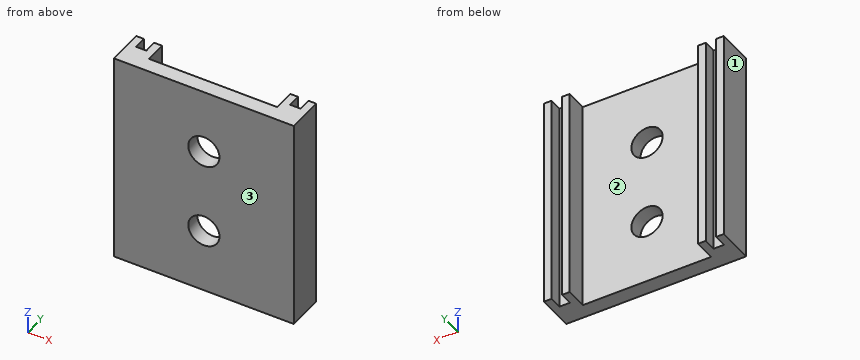
```python
from build123d import *

# Parameters (mm, degrees)
SKETCH1_W               = 40
SKETCH1_H               = 50
BOSS_EXTRUDE1_DEPTH     = 3.5
SKETCH2_W               = 40
SKETCH2_H               = 4
BOSS_EXTRUDE2_DEPTH     = 5
SKETCH3_W               = 4
SKETCH3_H               = 46
BOSS_EXTRUDE3_DEPTH     = 5
SKETCH4_W               = 2.4
SKETCH4_H               = 50
CUT_EXTRUDE1_DEPTH      = 3
SKETCH18_W              = 50
SKETCH18_H              = 8.5
BOSS_EXTRUDE8_DEPTH     = 1
SKETCH19_R              = 3.65
CUT_EXTRUDE2_DEPTH      = 6
CUT_EXTRUDE2_DEPTH_BACK = 4.5
SKETCH20_W              = 32
SKETCH20_H              = 4
CUT_EXTRUDE3_DEPTH      = 5
SKETCH21_W              = 50
SKETCH21_H              = 5
BOSS_EXTRUDE9_DEPTH     = 1


with BuildPart() as part:
    # Sketch1 → Boss-Extrude1 (new body)
    with BuildSketch(Plane(origin=(0, 0, 0), x_dir=(1, 0, 0), z_dir=(0, 1, 0))):
        Rectangle(SKETCH1_W, SKETCH1_H)
    extrude(amount=BOSS_EXTRUDE1_DEPTH)

    # Sketch2 → Boss-Extrude2 (add)
    with BuildSketch(Plane(origin=(0, 3.5, 0), x_dir=(1, 0, 0), z_dir=(0, 1, 0))):
        with Locations((0, 23)):
            Rectangle(SKETCH2_W, SKETCH2_H)
    extrude(amount=BOSS_EXTRUDE2_DEPTH)

    # Sketch3 → Boss-Extrude3 (add)
    with BuildSketch(Plane(origin=(0, 3.5, 0), x_dir=(1, 0, 0), z_dir=(0, 1, 0))):
        with Locations((-18, -2)):
            Rectangle(SKETCH3_W, SKETCH3_H)
    boss_extrude3 = extrude(amount=BOSS_EXTRUDE3_DEPTH)

    # Sketch4 → Cut-Extrude1 (cut)
    with BuildSketch(Plane(origin=(0, 8.5, 0), x_dir=(1, 0, 0), z_dir=(0, 1, 0))):
        with Locations((-18, 0)):
            Rectangle(SKETCH4_W, SKETCH4_H)
    cut_extrude1 = extrude(amount=-CUT_EXTRUDE1_DEPTH, mode=Mode.SUBTRACT)

    # Mirror1: Boss-Extrude3, Cut-Extrude1 across plane
    add(boss_extrude3.mirror(Plane(origin=(0, 0, 0), x_dir=(0, 0, 1), z_dir=(1, 0, 0))))
    add(cut_extrude1.mirror(Plane(origin=(0, 0, 0), x_dir=(0, 0, 1), z_dir=(1, 0, 0))), mode=Mode.SUBTRACT)

    # Sketch18 → Boss-Extrude8 (add)
    with BuildSketch(Plane.ZY.offset(20)):
        with Locations((0, 4.25)):
            Rectangle(SKETCH18_W, SKETCH18_H)
    boss_extrude8 = extrude(amount=BOSS_EXTRUDE8_DEPTH)

    # Mirror5: Boss-Extrude8 across plane
    add(boss_extrude8.mirror(Plane(origin=(0, 0, 0), x_dir=(0, 0, 1), z_dir=(1, 0, 0))))

    # Sketch19 → Cut-Extrude2 (cut, two sides)
    with BuildSketch(Plane(origin=(0, 3.5, 0), x_dir=(1, 0, 0), z_dir=(0, 1, 0))) as cut_extrude2_sk:
        with Locations((0, -10)):
            Circle(SKETCH19_R)
        with Locations((0, 10)):
            Circle(SKETCH19_R)
    extrude(amount=CUT_EXTRUDE2_DEPTH, mode=Mode.SUBTRACT)
    extrude(cut_extrude2_sk.sketch, amount=-CUT_EXTRUDE2_DEPTH_BACK, mode=Mode.SUBTRACT)

    # Sketch20 → Cut-Extrude3 (cut)
    with BuildSketch(Plane(origin=(0, 8.5, 0), x_dir=(1, 0, 0), z_dir=(0, 1, 0))):
        with Locations((0, 23)):
            Rectangle(SKETCH20_W, SKETCH20_H)
    extrude(amount=-CUT_EXTRUDE3_DEPTH, mode=Mode.SUBTRACT)

    # Sketch21 → Boss-Extrude9 (add)
    with BuildSketch(Plane(origin=(-16, 0, 0), x_dir=(0, 0, -1), z_dir=(1, 0, 0))):
        with Locations((0, 6)):
            Rectangle(SKETCH21_W, SKETCH21_H)
    boss_extrude9 = extrude(amount=BOSS_EXTRUDE9_DEPTH)

    # Mirror6: Boss-Extrude9 across plane
    add(boss_extrude9.mirror(Plane(origin=(0, 0, 0), x_dir=(0, 0, 1), z_dir=(1, 0, 0))))


solid = part.part
```
Check sheet for the modelled part. Datum: model origin and axes. Units: mm. Face numbers are marked on the shaded views. Coordinates: 2 decimals unless noted, no trailing zeros. Write each loop counter-clockwise with the first axis right and the second up, starting at its lowest first coordinate (ties: lowest second). Pieces come first, ordered by that corner, then holes. Notation, with made-up numbers: M 21.5,-7.75 L 43.5,-7.75 A31 ccw 43.5,25.25 Z; hole C 5.5,21.5 d11. An arc over 180 degrees is marked long. Use one line per item in the form item = value.
Item 1: Sectioned sample at A-A, the plane y = 6.25. Record the cut outline in (x, z).
Answer below:
outline = M -21,-25 L -19.2,-25 L -19.2,25 L -21,25 Z; M -16.8,-25 L -15,-25 L -15,25 L -16.8,25 Z; M 15,-25 L 16.8,-25 L 16.8,25 L 15,25 Z; M 19.2,-25 L 21,-25 L 21,25 L 19.2,25 Z
Item 2: Sectioned sample at D-D, the plane y = 2.75. Record the cut outline in (x, z), and give its area (3 significant figures).
Answer below:
outline = M -21,-25 L 21,-25 L 21,25 L -21,25 Z; hole C 0,-10 d7.3; hole C 0,10 d7.3
area = 2,020 mm^2
Item 3: Release check for a two-part mould opening along X. For the marked faces 1, 2 and 3 record: pulls with the +X half, pulls with the -X half, needs draft (parallel to the pull), parting line crosses it, or undercut.
Answer below:
face_1 = pulls with the -X half
face_2 = undercut
face_3 = needs draft
Item 4: Sectioned sample at C-C, the plane x = 0. Record the cut outline in (y, z), and give its area (3 significant figures).
Answer below:
outline = M 0,-25 L 3.5,-25 L 3.5,-13.65 L 0,-13.65 Z; M 0,-6.35 L 3.5,-6.35 L 3.5,6.35 L 0,6.35 Z; M 0,13.65 L 3.5,13.65 L 3.5,25 L 0,25 Z
area = 124 mm^2
Item 5: Sectioned sample at B-B, the plane z = 10. Record the cut outline in (x, y), and give its area (3 significant figures).
Answer below:
outline = M -21,0 L -3.65,0 L -3.65,3.5 L -15,3.5 L -15,8.5 L -16.8,8.5 L -16.8,5.5 L -19.2,5.5 L -19.2,8.5 L -21,8.5 Z; M 3.65,0 L 21,0 L 21,8.5 L 19.2,8.5 L 19.2,5.5 L 16.8,5.5 L 16.8,8.5 L 15,8.5 L 15,3.5 L 3.65,3.5 Z
area = 167 mm^2
Item 6: Material ranges on L1, parallel to X at y = 6.25, z = 20; L2, parallel to Z at x = 0, y = 1.15; L3, parallel to Z at x = 2, y = 2, recorded low to high. Write a range as from..to.
Answer below:
L1 = -21..-19.2, -16.8..-15, 15..16.8, 19.2..21
L2 = -25..-13.65, -6.35..6.35, 13.65..25
L3 = -25..-13.05, -6.95..6.95, 13.05..25
Item 7: Gauge pin test, flat ends, axial feed: pin 1 Ø4 at (x, y) = (2, 7) entering from -Z; pin 2 Ø1.2 at (x, z) = (18.5, -2.5) entering from +Y; pin 3 Ø8.5 at (x, z) = (0, -10) entering from +Y. Record the tip position at first contact, or that the pin passes through.
Answer below:
pin_1 = through
pin_2 = 5.5
pin_3 = 3.5
